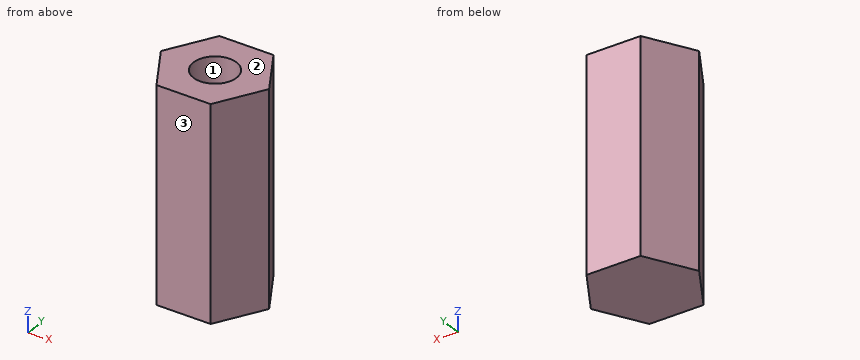
Autodesk Inventor part; units mm, degrees
ref_plane "YZ Plane" through (0, 0, 0) normal (1, 0, 0) x (0, 1, 0)
ref_plane "XZ Plane" through (0, 0, 0) normal (0, 1, 0) x (-1, 0, 0)
ref_plane "XY Plane" through (0, 0, 0) normal (0, 0, 1) x (1, 0, 0)
sketch "Sketch1" plane through (0, 0, 0) normal (0, 0, 1) x (1, 0, 0)
  line L0 (4.0415, 0) -> (2.0207, -3.5)
  line L1 (2.0207, -3.5) -> (-2.0207, -3.5)
  line L2 (-2.0207, -3.5) -> (-4.0415, 0)
  line L3 (-4.0415, 0) -> (-2.0207, 3.5)
  line L4 (-2.0207, 3.5) -> (2.0207, 3.5)
  line L5 (2.0207, 3.5) -> (4.0415, 0)
  point P0 (0, 0)
  point P1 (0, 0)
  dimension "d0" = 7
extrude "Extrusion1" add sketch "Sketch1" along normal blind 16
sketch "Sketch2" plane through (0, 0, 16) normal (0, 0, 1) x (1, 0, 0)
  point P0 (0, 0)
  point P1 (0, 0)
hole "Hole1" at (0, 0, 16) direction (0, 0, -1) diameter 3.242 depth 11.8
properties part number "magneet stand-offs16 mm"
Geometry check sheet. Reference: the model listing, model coordinates, mm. Face numbers are marked on the shaded views. Coordinates: 2 decimals unless noted, no trailing zeros. Order: outer loops, then holes, each group sorted by start corner. A loop starts at its lowest first (then second) coordinate and runs counter-clockwise, first axis right, second up. Notation, with made-up numbers: M -13.75,55.25 L 13.25,55.25 A9 ccw 13.25,61.25 Z; hole C 33.5,82.25 d6. An arc over 180 degrees is marked long. One line per question, with ' | ' between items. Start each with the question number.
Item 1: Gauge pin test, flat ends, axial feed: pin 1 (1.5 mm diameter, centred on y = -1.5, z = 7, fed in from +X); pin 2 (3 mm diameter, centred on y = 2.5, z = 12.5, fed in from -X). Record the tip position at first contact, or that the pin passes through.
Item 2: Draft check along Y on the marked faces 1, 2 and 3. Enter one of: pulls with the +Y half, pulls with the -Y half, needs draft (parallel to the pull), parting line crosses it, or undercut.
Item 3: Cross-section at C-C on x = 0. Enter the section's corners in (y, z), then the cut area to 3 significant figures.
Item 4: Cross-section at B-B on y = 1. Enter the section's corners in (x, z), then the cut area to 3 significant figures.
Item 5: Cross-section at D-D on x = 3. Enter the section's corners in (y, z).
Item 6: Cross-section at A-A on z = 10. Enter the section's corners in (x, y), then the cut area to 3 significant figures.
Item 7: Material ranges on L1, parallel to Y at x = 0, z = 11; L2, parallel to Z at x = 0.25, y = -0.5; L3, parallel to X at y = 1.75, z = 3.75, recorded low to high. Write a range as [from, to].
Findings:
1) pin 1: stops at x = 3.61 | pin 2: stops at x = -3.46
2) face 1: undercut | face 2: needs draft | face 3: pulls with the -Y half
3) outline: M -3.5,0 L 3.5,0 L 3.5,16 L 1.62,16 L 1.62,4.2 L -1.62,4.2 L -1.62,16 L -3.5,16 Z | area: 73.7 mm²
4) outline: M -3.46,0 L 3.46,0 L 3.46,16 L 1.28,16 L 1.28,4.2 L -1.28,4.2 L -1.28,16 L -3.46,16 Z | area: 80.7 mm²
5) outline: M -1.8,0 L 1.8,0 L 1.8,16 L -1.8,16 Z
6) outline: M -4.04,0 L -2.02,-3.5 L 2.02,-3.5 L 4.04,0 L 2.02,3.5 L -2.02,3.5 Z; hole C 0,0 d3.24 | area: 34.2 mm²
7) L1: y = [-3.5, -1.62], [1.62, 3.5] | L2: z = [0, 4.2] | L3: x = [-3.03, 3.03]
